Input: dimensioned drawing with shaded views. Units: mm. Origin: part minimum x, y, z. A direction names the side the tool comes from. Round coordinates to 2 decimals unless told otherwise and drop trailing zeros. Loops run counter-clockwise (first coordinate to the right, second up) from the corner with the lowest first, then second, coordinate; pieces in that order, holes last. Notation, with made-up numbers: (26.25, 39.5) - (69.25, 39.5) arc R20 cw to (69.25, 77.5) - close; hole circle Ø4 at (16.25, 46). An arc over 180 degrees is marked (long way). One line per question, with ' | ' between items.
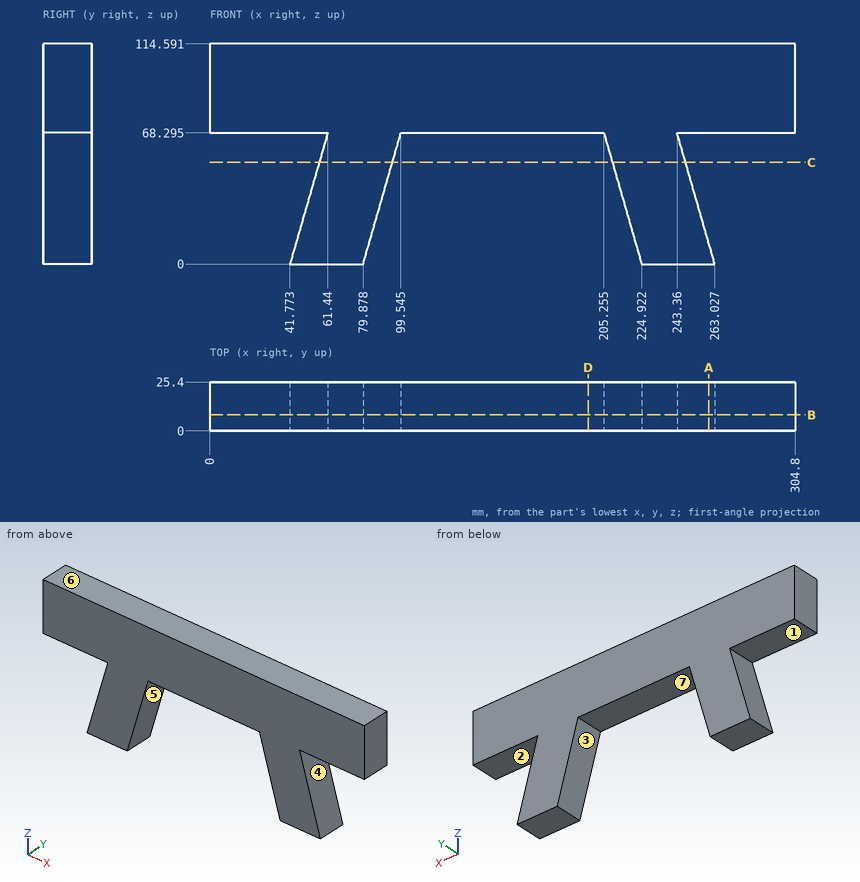
1. Material intervals for probe 1 along X at (y, z) = (18.25, 64); probe 2 along X at (y, z) = (14.75, 40.5) (1 decimal); probe 3 along Z at (x, y) = (119, 10.25) (1 decimal), sorted ascending.
Worked out:
probe 1: x = 60.2 to 98.31, 206.49 to 244.6 | probe 2: x = 53.4 to 91.5, 213.3 to 251.4 | probe 3: z = 68.3 to 114.6
2. Section query D-D, the plane x = 197. Return loops of the section in (y, z) (1 decimal).
Worked out:
outline: (0, 68.3) - (25.4, 68.3) - (25.4, 114.6) - (0, 114.6) - close
3. Access query for the marked faces 1, 2 and 3. Directions: +Z, -Z, +X, -X, +Y, -Y. A direction counts if a zero-diameter tool reaches every point of the face in a straight line with its end or side. Return the directions, or none.
Worked out:
face 1: -X, +Y, -Y | face 2: +X, +Y, -Y | face 3: -Z, +Y, -Y
4. Section query A-A, the plane x = 260. Return loops of the section in (y, z) (1 decimal), plus the area to 3 significant figures.
Worked out:
outline: (0, 0) - (25.4, 0) - (25.4, 10.5) - (0, 10.5) - close; (0, 68.3) - (25.4, 68.3) - (25.4, 114.6) - (0, 114.6) - close | area: 1,440 mm2
5. Contact query for flat-ended pins moving along their axis: P1, Ø12.5, axis at x = 34.5, y = 19, coming from the -Z side (1 decimal); P2, Ø2, axis at x = 261, y = 22.5, coming from the -Z side; P3, Ø4, axis at y = 23, z = 56, coming from the +X side; P4, Ø3, axis at y = 17, z = 36.5, coming from the -X side. Output: stop coordinate, or through.
Worked out:
P1: stops at z = 68.3 | P2: stops at z = 0 | P3: stops at x = 247.48 | P4: stops at x = 51.85
6. Section query C-C, the plane z = 53. Return loops of the section in (x, y) (1 decimal), plus the area to 3 significant figures.
Worked out:
outline: (57, 0) - (95.1, 0) - (95.1, 25.4) - (57, 25.4) - close; (209.7, 0) - (247.8, 0) - (247.8, 25.4) - (209.7, 25.4) - close | area: 1,940 mm2
7. Section query B-B, the plane y = 8.25. Return loops of the section in (x, z) (1 decimal).
Worked out:
outline: (0, 68.3) - (61.4, 68.3) - (41.8, 0) - (79.9, 0) - (99.5, 68.3) - (205.3, 68.3) - (224.9, 0) - (263, 0) - (243.4, 68.3) - (304.8, 68.3) - (304.8, 114.6) - (0, 114.6) - close
8. Mould query, pull axis X, two halves, no side actions, for the marked faces 4, 5, 6 and 7. Classes: released by +X, released by -X, zero draft, split by the parting line, or undercut.
Worked out:
face 4: released by +X | face 5: undercut | face 6: zero draft | face 7: undercut
